```python
from build123d import *

# Parameters (mm, degrees)
F1_DEPTH = 6.35
F3_DEPTH = 25.4
F5_DEPTH = 25.4


with BuildPart() as f1:
    # F0 (on Top) → F1 (new body)
    with BuildSketch(Plane.XY):
        with BuildLine():
            Line((118.2751, 84.1375), (-118.2751, 84.1375))
            ThreePointArc((-118.2751, 84.1375), (-118.831876, 83.906876), (-119.0625, 83.3501))
            Line((-119.0625, 83.3501), (-119.0625, -83.3501))
            ThreePointArc((-119.0625, -83.3501), (-118.831876, -83.906876), (-118.2751, -84.1375))
            Line((-118.2751, -84.1375), (118.2751, -84.1375))
            ThreePointArc((118.2751, -84.1375), (118.831876, -83.906876), (119.0625, -83.3501))
            Line((119.0625, -83.3501), (119.0625, 83.3501))
            ThreePointArc((119.0625, 83.3501), (118.831876, 83.906876), (118.2751, 84.1375))
        make_face()
    extrude(amount=F1_DEPTH)

    # F2 (on face) → F3 (cut)
    with BuildSketch(Plane.XY.offset(6.35)):
        Polygon((-2.690393, 31.790107), (-65.682393, 31.790107), (-97.4725, 0), (-65.682393, -31.790107), (61.825607, -31.790107), (93.615713, 0), (29.099713, 0), align=None)
    extrude(amount=-F3_DEPTH, mode=Mode.SUBTRACT)

    # F4 (on face) → F5 (cut)
    with BuildSketch(Plane.XY.offset(6.35)):
        with BuildLine():
            ThreePointArc((29.951916, 1.27), (29.650591, 1.329937), (29.39514, 1.500624))
            Line((29.39514, 1.500624), (-1.933718, 32.829483))
            ThreePointArc((-1.933718, 32.829483), (-2.189169, 33.000169), (-2.490494, 33.060107))
            Line((-2.490494, 33.060107), (-65.882293, 33.060107))
            ThreePointArc((-65.882293, 33.060107), (-66.183618, 33.000169), (-66.439069, 32.829483))
            Line((-66.439069, 32.829483), (-98.711775, 0.556776))
            ThreePointArc((-98.711775, 0.556776), (-98.942399, 0), (-98.711775, -0.556776))
            Line((-98.711775, -0.556776), (-66.439069, -32.829483))
            ThreePointArc((-66.439069, -32.829483), (-66.183618, -33.000169), (-65.882293, -33.060107))
            Line((-65.882293, -33.060107), (62.025506, -33.060107))
            ThreePointArc((62.025506, -33.060107), (62.326831, -33.000169), (62.582282, -32.829483))
            Line((62.582282, -32.829483), (95.337589, -0.074176))
            ThreePointArc((95.337589, -0.074176), (95.508276, 0.783925), (94.780813, 1.27))
            Line((94.780813, 1.27), (29.951916, 1.27))
        make_face()
    extrude(amount=-F5_DEPTH, mode=Mode.SUBTRACT)


solid = f1.part
```
Geometry check sheet. Reference: the model listing, model coordinates, mm. A direction names the side the tool comes from. Round coordinates to 2 decimals unless told otherwise and drop trailing zeros. Order: outer loops, then holes, each group sorted by start corner. A loop starts at its lowest first (then second) coordinate and runs counter-clockwise, first axis right, second up. Notation, with made-up numbers: M 0.5,66 L 32.5,66 A16 cw 32.5,70 Z; hole C 29.25,22.25 d4. An arc over 180 degrees is marked long. Write item = value, one per line.
Q1. Scan lines: line 1 (Y direction, x = 61.5, z = 4.5); line 2 (Y direction, x = -46, z = 6); line 3 (X direction, y = 18, z = 3). Record each from-to range of solid material in increasing order.
Answer block:
line_1 = -84.14 to -33.06, 1.27 to 84.14
line_2 = -84.14 to -33.06, 33.06 to 84.14
line_3 = -119.06 to -81.27, 12.9 to 119.06
Q2. Set-up check for faces 1 (the flat face through (-2, -84.138, 3)), 2 (the flat face through (-3, -33.06, 3)): record each of +Z, -Z, +X, -X, +Y, -Y from which the full face is reachable in a straight line by a thin tool's end or side.
Answer block:
face_1 = +Z, -Z, +X, -X, -Y
face_2 = +Z, -Z
Q3. Section check B-B (x = -16.5). Enter the section's corners in (y, z).
Answer block:
outline = M -84.14,0 L -33.06,0 L -33.06,6.35 L -84.14,6.35 Z; M 33.06,0 L 84.14,0 L 84.14,6.35 L 33.06,6.35 Z
Q4. Release check for a two-part mould opening along Y. For faces 3 (the flat face through (13.95, 16.946, 3.219)), 4 (the flat face through (-119.062, 1, 3)), 5 (the flat face through (-82.35, 16.92, 3.22)), 6 (the flat face through (2, 84.138, 3)) record: released by +Y, released by -Y, zero draft, split by the parting line, or undercut.
Answer block:
face_3 = undercut
face_4 = zero draft
face_5 = undercut
face_6 = released by +Y
Q5. Section check A-A (z = 1.5). Enter the section's corners in (x, y) (1 decimal), plus the area to 3 significant figures.
Answer block:
outline = M -119.1,-83.4 A0.8 ccw -118.3,-84.1 L 118.3,-84.1 A0.8 ccw 119.1,-83.4 L 119.1,83.4 A0.8 ccw 118.3,84.1 L -118.3,84.1 A0.8 ccw -119.1,83.4 Z; hole M -98.7,-0.6 L -66.4,-32.8 A0.8 ccw -65.9,-33.1 L 62,-33.1 A0.8 ccw 62.6,-32.8 L 95.3,-0.1 A0.8 ccw 94.8,1.3 L 30,1.3 A0.8 cw 29.4,1.5 L -1.9,32.8 A0.8 ccw -2.5,33.1 L -65.9,33.1 A0.8 ccw -66.4,32.8 L -98.7,0.6 A0.8 ccw Z
area = 31,400 mm^2
Q6. Section check C-C (y = 13.5). Enter the section's corners in (x, z), plus the area to 3 significant figures.
Answer block:
outline = M -119.06,0 L -85.77,0 L -85.77,6.35 L -119.06,6.35 Z; M 17.4,0 L 119.06,0 L 119.06,6.35 L 17.4,6.35 Z
area = 857 mm^2
